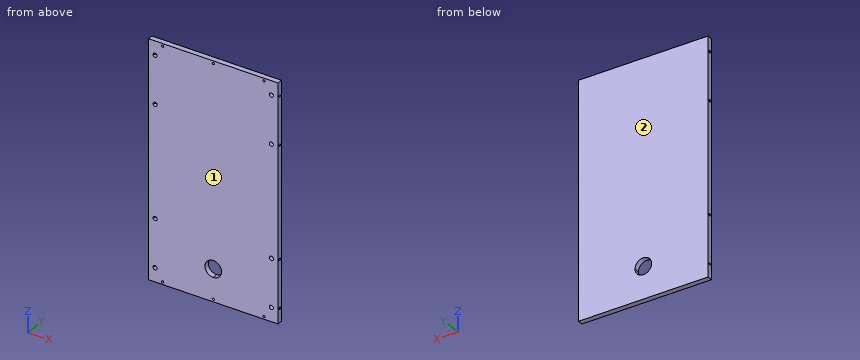
```python
from build123d import *

# Parameters (mm, degrees)
F0_W     = 469.9
F0_H     = 857.25
F1_DEPTH = 19.05
F3_D     = 8.001
F3_DEPTH = 14.224
F3_TIP   = 2.4037429064
F5_D     = 15.0114
F5_DEPTH = 14.224
F5_TIP   = 4.5098795482
F7_D     = 8.001
F7_DEPTH = 25.4
F7_TIP   = 2.4037429064
F9_D     = 8.001
F9_DEPTH = 25.4
F9_TIP   = 2.4037429064


with BuildPart() as f1:
    # F0 (on Front) → F1 (new body)
    with BuildSketch(Plane.XZ):
        Rectangle(F0_W, F0_H)
        with BuildLine():
            ThreePointArc((0, -341.8299634457), (-21.3281082875, -290.3393551581), (30.1625, -311.6674634457))
            ThreePointArc((30.1625, -311.6674634457), (21.3281082875, -332.9955717332), (0, -341.8299634457))
        make_face(mode=Mode.SUBTRACT)
    extrude(amount=F1_DEPTH)

    # F3
    with Locations(Plane.XZ.offset(19.05)):
        with Locations((-184.15, 419.1), (0, 419.1), (184.15, 419.1), (-184.15, -419.1), (0, -419.1), (184.15, -419.1)):
            Hole(F3_D / 2, depth=F3_DEPTH)
            with Locations((0, 0, -(F3_DEPTH + F3_TIP / 2))):  # 118° drill point
                Cone(0, F3_D / 2, F3_TIP, mode=Mode.SUBTRACT)

    # F5
    with Locations(Plane.XZ.offset(19.05)):
        with Locations((-211.074, 377.825), (211.074, 377.825), (211.074, 203.2), (-211.074, 203.2), (-211.074, -203.2), (211.074, -203.2), (211.074, -377.825), (-211.074, -377.825)):
            Hole(F5_D / 2, depth=F5_DEPTH)
            with Locations((0, 0, -(F5_DEPTH + F5_TIP / 2))):  # 118° drill point
                Cone(0, F5_D / 2, F5_TIP, mode=Mode.SUBTRACT)

    # F7
    with Locations(Plane.YZ.offset(234.95)):
        with Locations((-9.525, 377.825), (-9.525, 203.2), (-9.525, -203.2), (-9.525, -377.825)):
            Hole(F7_D / 2, depth=F7_DEPTH)
            with Locations((0, 0, -(F7_DEPTH + F7_TIP / 2))):  # 118° drill point
                Cone(0, F7_D / 2, F7_TIP, mode=Mode.SUBTRACT)

    # F9
    with Locations(Plane(origin=(-234.95, 0, 0), x_dir=(0, -1, 0), z_dir=(-1, 0, 0))):
        with Locations((9.525, 377.825), (9.525, 203.2), (9.525, -203.2), (9.525, -377.825)):
            Hole(F9_D / 2, depth=F9_DEPTH)
            with Locations((0, 0, -(F9_DEPTH + F9_TIP / 2))):  # 118° drill point
                Cone(0, F9_D / 2, F9_TIP, mode=Mode.SUBTRACT)


solid = f1.part
```
Input: part model. Units: mm. Frame: model coordinates. Face numbers are marked on the shaded views. Round coordinates to 2 decimals unless told otherwise and drop trailing zeros. Answer as CSV lines item,"result".
1. Contact query for flat-ended pins moving along their axis: P1, Ø9, axis at x = 184.15, z = -419.1, coming from the -Y side; P2, Ø13.5, axis at x = 211.074, z = -203.2, coming from the -Y side; P3, Ø5, axis at y = -9.525, z = -203.2, coming from the +X side; P4, Ø7, axis at y = -9.525, z = -203.2, coming from the +X side. Output: stop coordinate, or through.
Geometry says:
P1,"stops at y = -19.05"
P2,"stops at y = -4.37"
P3,"stops at x = 204"
P4,"stops at x = 204.43"
2. Mould query, pull axis Y, two halves, no side actions, for the marked faces 1 and 2. Classes: +Y half, -Y half, draft (parallel to the pull), parting line (faces both ways), or undercut.
Geometry says:
face 1,"-Y half"
face 2,"+Y half"
3. Ray query, L1, parallel to Z at x = -184.15, y = -14.75 (1 decimal); L2, parallel to X at y = -8.5, z = 419.1; L3, parallel to Z at x = 207.5, y = -6.25 (3 decimals). Return the intervals inside material, ascending. Write a range as [from, to].
Geometry says:
L1,"z = [-428.6, -423.1], [-415.1, 415.1], [423.1, 428.6]"
L2,"x = [-234.95, -188.15], [-180.15, -4], [4, 180.15], [188.15, 234.95]"
L3,"z = [-428.625, -384.425], [-371.225, -209.8], [-196.6, 196.6], [209.8, 371.225], [384.425, 428.625]"
